Geometry: see drawing. Coordinates: mm, zero at the bounding-box minimum. A direction names the side the tool comes from. Round coordinates to 2 decimals unless told otherwise and drop trailing zeros. Order: outer loops, then holes, each group sorted by start corner. A loop starts at its lowest first (then second) coordinate and runs counter-clockwise, first axis right, second up. Notation, with made-up numbers: (26, 70.25) -> (40, 70.25) arc R17 ccw to (40, 101.25) -> close; hole circle Ø11 at (37.25, 11.25). An arc over 180 degrees is marked (long way). Put each result on its own line as item: value.
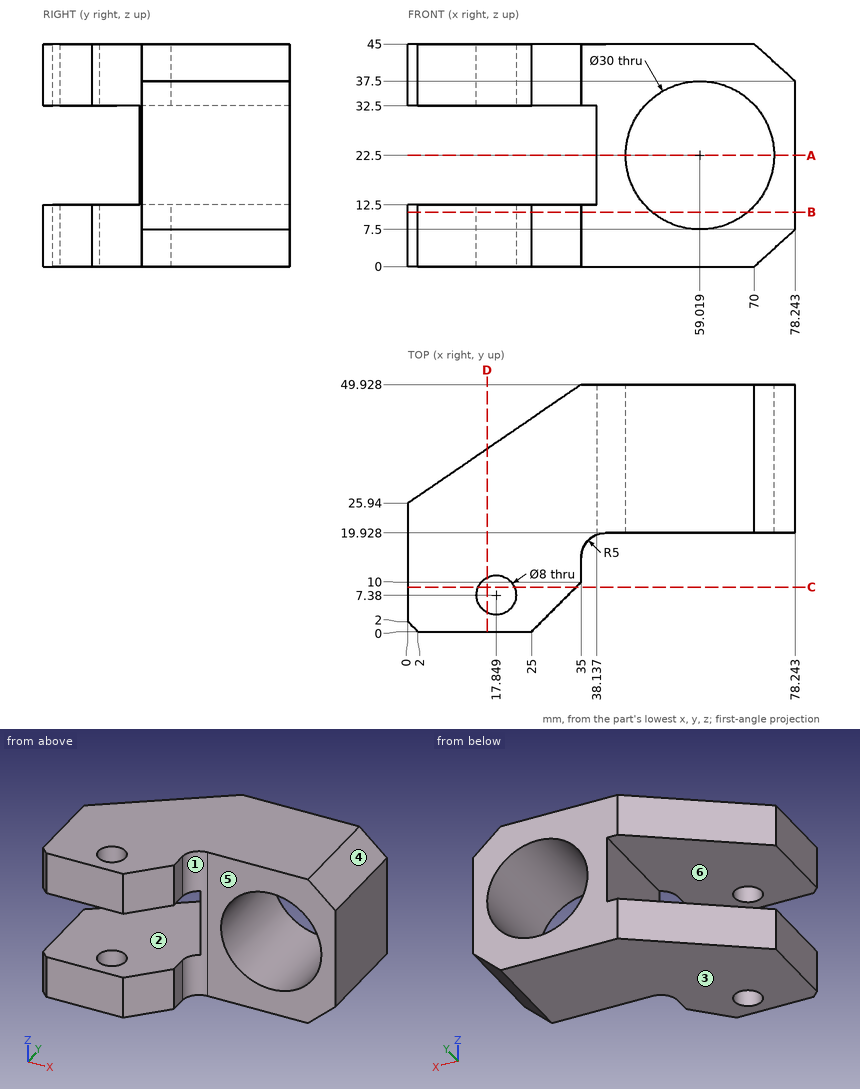
1. Cut plane A-A on z = 22.5. Return loops of the section in (x, y).
Ans:
outline: (38.14, 19.57) arc R5 cw to (40, 19.93) -> (44.02, 19.93) -> (44.02, 49.93) -> (38.14, 49.93) -> close; (74.02, 19.93) -> (78.24, 19.93) -> (78.24, 49.93) -> (74.02, 49.93) -> close
2. Cut plane B-B on z = 11. Return loops of the section in (x, y).
Ans:
outline: (0, 2) -> (2, 0) -> (25, 0) -> (35, 10) -> (35, 14.93) arc R5 cw to (40, 19.93) -> (49.39, 19.93) -> (49.39, 49.93) -> (35, 49.93) -> (0, 25.94) -> close; (68.65, 19.93) -> (78.24, 19.93) -> (78.24, 49.93) -> (68.65, 49.93) -> close; hole circle Ø8 at (17.85, 7.38)
3. Draft query along Z for the marked faces 1, 2 and 3. Return one class per face: +Z half, -Z half, draft (parallel to the pull), parting line (faces both ways), or undercut.
Ans:
face 1: draft
face 2: undercut
face 3: -Z half
4. Contact query for flat-ended pins moving along their axis: P1, Ø1.5, axis at x = 17, y = 34, coming from the -Z side; P2, Ø2.5, axis at y = 12, z = 39, coming from the +X side; P3, Ø2, axis at y = 40.5, z = 20, coming from the -X side; P4, Ø19, axis at x = 66, z = 14, coming from the -Y side. Output: stop coordinate, or through.
Ans:
P1: z = 0
P2: x = 35
P3: x = 38.14
P4: y = 19.93
5. Set-up query: the marked faces 4, 5 and 6. Return all of +Z, -Z, +X, -X, +Y, -Y with unobstructed straight access to the full face (end or side cutting, diameter ignored); none if empty.
Ans:
face 4: +Z, +X, +Y, -Y
face 5: +Z, -Z, +X, -Y
face 6: -X, +Y, -Y
6. Material intervals for probe 1 along X at (y, z) = (41, 22.5); probe 2 along Z at (x, y) = (23.5, 17); probe 3 along Y at (x, z) = (72.5, 9), sorted ascending.
Ans:
probe 1: 38.14 to 44.02, 74.02 to 78.24
probe 2: 0 to 12.5, 32.5 to 45
probe 3: 19.93 to 49.93
7. Cut plane C-C on y = 9. Return loops of the section in (x, z) (1 decimal).
Ans:
outline: (0, 0) -> (14.2, 0) -> (14.2, 12.5) -> (0, 12.5) -> close; (0, 32.5) -> (14.2, 32.5) -> (14.2, 45) -> (0, 45) -> close; (21.5, 0) -> (34, 0) -> (34, 12.5) -> (21.5, 12.5) -> close; (21.5, 32.5) -> (34, 32.5) -> (34, 45) -> (21.5, 45) -> close
8. Cut plane D-D on x = 16. Return loops of the section in (y, z) (1 decimal).
Ans:
outline: (0, 0) -> (3.8, 0) -> (3.8, 12.5) -> (0, 12.5) -> close; (0, 32.5) -> (3.8, 32.5) -> (3.8, 45) -> (0, 45) -> close; (10.9, 0) -> (36.9, 0) -> (36.9, 12.5) -> (10.9, 12.5) -> close; (10.9, 32.5) -> (36.9, 32.5) -> (36.9, 45) -> (10.9, 45) -> close
